```python
from build123d import *
from OCP.BRepFilletAPI import BRepFilletAPI_MakeChamfer

# Parameters (mm, degrees)
BOSS_EXTRUDE1_DEPTH = 7.9
SKETCH2_R           = 1.5
CUT_EXTRUDE1_DEPTH  = 52.15085532
CUT_EXTRUDE3_DEPTH  = 3
BOSS_EXTRUDE2_DEPTH = 3
SKETCH5_W           = 8.304797865
SKETCH5_H           = 8.5
CUT_EXTRUDE4_DEPTH  = 49.408780195
CHAMFER1_SIZE       = 2
CHAMFER1_SIZE2      = 3.079729928


with BuildPart() as part:
    # Sketch1 → Boss-Extrude1 (new body)
    with BuildSketch(Plane.XY):
        Polygon((30, 8), (30, 0), (22, 0), (22, -7), (33.5, -7), (45, 4.5), (45, 16), (38, 16), (38, 8), align=None)
    extrude(amount=-BOSS_EXTRUDE1_DEPTH)

    # Sketch2 → Cut-Extrude1 (cut, through all)
    with BuildSketch(Plane.XZ.offset(7)):
        with Locations((27, -3.95)):
            Circle(SKETCH2_R)
    cut_extrude1 = extrude(amount=-CUT_EXTRUDE1_DEPTH, mode=Mode.SUBTRACT)

    # Sketch3 → Cut-Extrude3 (cut)
    with BuildSketch(Plane(origin=(38, -7, 0), x_dir=(0, 0, -1), z_dir=(0, 1, 0))):
        Polygon((0.95, 12.732050808), (3.95, 14.464101615), (6.95, 12.732050808), (6.95, 9.267949192), (3.95, 7.535898385), (0.95, 9.267949192), align=None)
    cut_extrude3 = extrude(amount=CUT_EXTRUDE3_DEPTH, mode=Mode.SUBTRACT)

    # Sketch4 → Boss-Extrude2 (add)
    with BuildSketch(Plane.XY):
        Polygon((22, 0), (38, 16), (45, 16), (45, 4.5), (33.5, -7), (22, -7), align=None)
    extrude(amount=BOSS_EXTRUDE2_DEPTH)

    # Sketch5 → Cut-Extrude4 (cut, through all)
    with BuildSketch(Plane(origin=(0, 0, 0), x_dir=(1, 0, 0), z_dir=(0, 1, 0))):
        with Locations((26.152398932, 3.95)):
            Rectangle(SKETCH5_W, SKETCH5_H)
    cut_extrude4 = extrude(amount=CUT_EXTRUDE4_DEPTH, mode=Mode.SUBTRACT)

    # Mirror1: Cut-Extrude1, Cut-Extrude3, Cut-Extrude4 across plane
    add(cut_extrude1.mirror(Plane(origin=(19, 19, 0), x_dir=(0, 0, 1), z_dir=(0.707106781186547, 0.707106781186548, 0))), mode=Mode.SUBTRACT)
    add(cut_extrude3.mirror(Plane(origin=(19, 19, 0), x_dir=(0, 0, 1), z_dir=(0.707106781186547, 0.707106781186548, 0))), mode=Mode.SUBTRACT)
    add(cut_extrude4.mirror(Plane(origin=(19, 19, 0), x_dir=(0, 0, 1), z_dir=(0.707106781186547, 0.707106781186548, 0))), mode=Mode.SUBTRACT)

    # Chamfer1: one chamfer whose edges measure the first distance from different faces: ONE call of the kernel's chamfer builder (chamfer() names one face for all edges)
    chamfer1_edges_1 = [part.edges().sort_by_distance(p)[0] for p in [
        (34.152398932, 7.695202135, -7.9),
    ]]
    chamfer1_side_1 = [part.faces().sort_by_distance(p)[0] for p in [
        (34.152398932, 7.695202135, -3.8),
    ]]
    chamfer1_edges_2 = [part.edges().sort_by_distance(p)[0] for p in [
        (30.304797865, 3.847601068, -7.9),
    ]]
    chamfer1_side_2 = [part.faces().sort_by_distance(p)[0] for p in [
        (30.304797865, 3.847601068, -3.8),
    ]]
    chamfer1 = BRepFilletAPI_MakeChamfer(part.part.solid().wrapped)
    for e in chamfer1_edges_1:
        chamfer1.Add(CHAMFER1_SIZE, CHAMFER1_SIZE2, e.wrapped, chamfer1_side_1[0].wrapped)  # the first distance lies on this face
    for e in chamfer1_edges_2:
        chamfer1.Add(CHAMFER1_SIZE, CHAMFER1_SIZE2, e.wrapped, chamfer1_side_2[0].wrapped)  # the first distance lies on this face
    add(Compound.cast(chamfer1.Shape()), mode=Mode.REPLACE)


solid = part.part
```
Could you check a few things on this model? Use its own coordinates, in mm. A direction names the side the tool comes from. Give positions to 0.01 mm unless a question says otherwise; leave off trailing zeros. Loops run counter-clockwise (first coordinate to the right, second up) from the corner with the lowest first, then second, coordinate; pieces in that order, holes last. Notation, with made-up numbers: (13.5, 70.25) - (20.5, 70.25) arc R19 cw to (20.5, 104.25) - close; hole circle Ø2 at (-36.5, 76). An arc over 180 degrees is marked (long way). Use one line per item in the form item = value.
1. I want a section at A-A (x = 27). Please give me the cut outline in (y, z), and give its area (3 significant figures).
Response values:
outline = (-7, -7.9) - (0, -7.9) - (0, -5.45) - (-4, -5.45) - (-4, -6.95) - (-7, -6.95) - close; (-7, -0.95) - (-4, -0.95) - (-4, -2.45) - (0, -2.45) - (0, 0.3) - (5, 0.3) - (5, 3) - (-7, 3) - close
area = 59.8 mm²
2. I want a section at C-C (z = 2.25). Please give me the cut outline in (x, y).
Response values:
outline = (22, -7) - (33.5, -7) - (45, 4.5) - (45, 16) - (38, 16) - (22, 0) - close
3. I need wall thicknesses on probe 1 along Z at (x, y) = (27, -2.45); probe 2 along Z at (x, y) = (29.75, 7.5); probe 3 along X at (y, z) = (1.5, -6). Which ranges of each line are inside material? Lowest first, please.
Response values:
probe_1 = -7.9 to -5.45, -2.45 to 3
probe_2 = 0.3 to 3
probe_3 = 30.46 to 42
4. Thinking about a two-plate mould opening in Y: for faces 4 (the face through (28.5, -4, -4.7)), 5 (the face through (30, 7, 0.3)), 6 (the face through (40.03, 9.57, -3.5)), 7 (the face through (34, 7.695, -3)), which applies, released by +Y, released by -Y, zero draft, split by the parting line, or undercut?
Response values:
face_4 = released by -Y
face_5 = zero draft
face_6 = undercut
face_7 = released by +Y
5. I want a section at B-B (y = 11). Please give me the cut outline in (x, z).
Response values:
outline = (33, 0.3) - (38, 0.3) - (38, -2.45) - (42, -2.45) - (42, -0.95) - (45, -0.95) - (45, 3) - (33, 3) - close; (38, -7.9) - (45, -7.9) - (45, -6.95) - (42, -6.95) - (42, -5.45) - (38, -5.45) - close
6. I want a section at D-D (x = 36). Please give me the cut outline in (y, z).
Response values:
outline = (-4.5, -7.9) - (4.62, -7.9) - (7.7, -5.9) - (7.7, 0.3) - (14, 0.3) - (14, 3) - (-4.5, 3) - close
7. On a 3-axis mill with a long thin cutter (end or side, diameter ignored), from which of +Z, -Z, +X, -X, +Y, -Y can I reach the whole of each face in a straight line? I mean faces 1 (the face through (30.305, 4, -3)), 2 (the face through (27, -6, -6.95)), 3 (the face through (43.521, 8.414, -5.471)). Say none if no direction works.
Response values:
face_1 = -Z, -X, +Y
face_2 = -Y
face_3 = +X
8. I'm going to push flat-ended pins straight in: pin 1 Ø1.5 at (x, z) = (34, -1.5) entering from +Y; pin 2 Ø5 at (x, y) = (27.5, 7.5) entering from -Z; pin 3 Ø2.5 at (y, z) = (11, -3.95) entering from +X; pin 4 Ø1.8 at (x, z) = (28, -3) entering from -Y. Where does each tip first touch, or does it pass through?
Response values:
pin_1 = 7.7
pin_2 = 0.3
pin_3 = through
pin_4 = -4
